Part model, mm, in its own coordinate system. A direction names the side the tool comes from. Give positions to 0.01 mm unless a question says otherwise; leave off trailing zeros. Order: outer loops, then holes, each group sorted by start corner. A loop starts at its lowest first (then second) coordinate and runs counter-clockwise, first axis right, second up. Notation, with made-up numbers: (5, 74.5) -> (43, 74.5) arc R14 ccw to (43, 83.5) -> close; hole circle Ø2 at (47, -29). An arc over 180 degrees is marked (long way). Write item = value, one per line. Start each with the question number.
Item 1: Drill centre lines: line 1 along Y through (x, z) = (-20.5, 11.5); line 2 along X through (y, z) = (-8, 0); line 3 along X through (y, z) = (-13, 1.5). Where is each one in solid material? Low to high.
Item 2: Tool access for faces 1 (the face through (21.2, 10, -7)), 2 (the face through (21.477, 16.986, 4.769)), 3 (the face through (21.477, -17.014, 4.769)): list every direction of +Z, -Z, +X, -X, +Y, -Y with a clear straight run to the whole face (end or side of a thin tool).
Item 3: Flat gauge pins, fed straight in: P1, Ø1.5, axis at y = 4.5, z = 11, coming from the -X side; P2, Ø5, axis at y = 8.5, z = -6.5, coming from the +X side; P3, Ø1, axis at y = -0.5, z = -3.5, coming from the -X side. Where does each tip first touch, or does it go through?
Item 4: Pull direction Y, two halves, no side cores. Call faces 4 (the face through (7, -10, 21.2)), 5 (the face through (21.2, -16, -7)), 6 (the face through (-7.21, -11.01, -22.89)): +Y half, -Y half, draft (parallel to the pull), parting line (faces both ways), or undercut.
Item 5: Band-saw the part on A-A on y = -6.5. Write the cut outline in (x, z).
```python
from build123d import *


with BuildPart() as part:
    # Esquisse1 → Révolution1 (revolve)
    with BuildSketch(Plane.XY, mode=Mode.PRIVATE) as r_volution1_sk:
        Polygon((22, 12), (24, 12), (24, 10), (22, 10), (22, -10), (24, -10), (24, -12), (22, -12), (22, -14), (24, -14), (24, -16), (22, -16), (22, -18), (11, -18), (11, 18), (22, 18), (22, 16), (24, 16), (24, 14), (22, 14), align=None)
    revolve(r_volution1_sk.sketch.rotate(Axis((0, 0, 0), (0, 1, 0)), 90), axis=Axis((0, 0, 0), (0, 1, 0)))


solid = part.part
```
Values found:
q1.line_1 = -16 to -14, -12 to -10, 10 to 12, 14 to 16
q1.line_2 = -22 to -11, 11 to 22
q1.line_3 = -21.95 to -10.9, 10.9 to 21.95
q2.face_1 = none
q2.face_2 = +Y
q2.face_3 = -Y
q3.P1 = -19.47
q3.P2 = 23.57
q3.P3 = -21.79
q4.face_4 = undercut
q4.face_5 = -Y half
q4.face_6 = draft
q5.outline = circle Ø44 at (0, 0); hole circle Ø22 at (0, 0)
